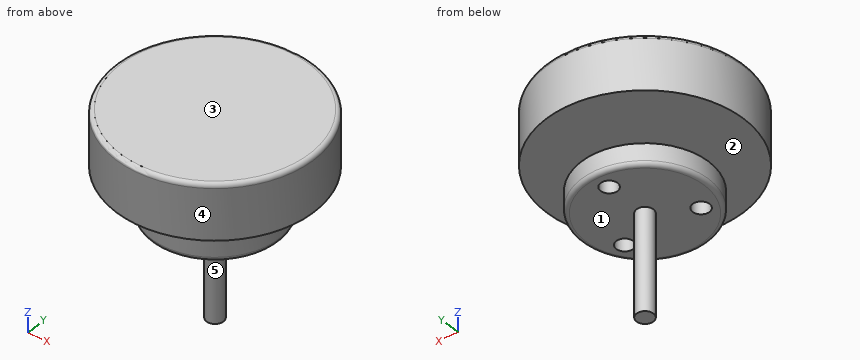
```python
from build123d import *

# Parameters (mm, degrees)
SKETCH1_R           = 11.65
BOSS_EXTRUDE1_DEPTH = 6.5
FILLET1_R           = 0.5
SKETCH2_R           = 3.25
BOSS_EXTRUDE2_DEPTH = 3
SKETCH3_R           = 7.5
BOSS_EXTRUDE3_DEPTH = 2.5
FILLET2_R           = 0.5
SKETCH4_R           = 1
BOSS_EXTRUDE4_DEPTH = 12
CUT_EXTRUDE1_REACH  = 22.382
SKETCH5_R           = 1


with BuildPart() as part:
    # Sketch1 → Boss-Extrude1 (new body)
    with BuildSketch(Plane.XY):
        with Locations(Location((0, 0, 0), (0, 0, 180))):
            Circle(SKETCH1_R)
    extrude(amount=BOSS_EXTRUDE1_DEPTH)

    # Fillet1
    fillet1_edges = [part.edges().sort_by_distance(p)[0] for p in [
        (11.65, 0, 6.5),
    ]]
    fillet(fillet1_edges, radius=FILLET1_R)

    # Sketch2 → Boss-Extrude2 (add)
    with BuildSketch(Plane(origin=(0, 0, 0), x_dir=(-1, 0, 0), z_dir=(0, 0, -1))):
        Circle(SKETCH2_R)
    extrude(amount=BOSS_EXTRUDE2_DEPTH)

    # Sketch3 → Boss-Extrude3 (add)
    with BuildSketch(Plane(origin=(0, 0, -3), x_dir=(-1, 0, 0), z_dir=(0, 0, -1))):
        Circle(SKETCH3_R)
    extrude(amount=BOSS_EXTRUDE3_DEPTH)

    # Fillet2
    fillet2_edges = [part.edges().sort_by_distance(p)[0] for p in [
        (7.5, 0, -5.5),
    ]]
    fillet(fillet2_edges, radius=FILLET2_R)

    # Sketch4 → Boss-Extrude4 (add)
    with BuildSketch(Plane(origin=(0, 0, -5.5), x_dir=(-1, 0, 0), z_dir=(0, 0, -1))):
        Circle(SKETCH4_R)
    extrude(amount=BOSS_EXTRUDE4_DEPTH)

    # Sketch5 → Cut-Extrude1 (cut, up to next)
    with BuildSketch(Plane(origin=(0, 0, -5.5), x_dir=(-1, 0, 0), z_dir=(0, 0, -1)), mode=Mode.PRIVATE) as cut_extrude1_sk1:
        with Locations((4.54663337, -2.625)):
            Circle(SKETCH5_R)
    cut_extrude1_tool1 = extrude(cut_extrude1_sk1.sketch, amount=-CUT_EXTRUDE1_REACH, mode=Mode.PRIVATE) & part.part
    # Sketch5 → Cut-Extrude1 (cut, up to next)
    with BuildSketch(Plane(origin=(0, 0, -5.5), x_dir=(-1, 0, 0), z_dir=(0, 0, -1)), mode=Mode.PRIVATE) as cut_extrude1_sk2:
        with Locations((0, 5.25)):
            Circle(SKETCH5_R)
    cut_extrude1_tool2 = extrude(cut_extrude1_sk2.sketch, amount=-CUT_EXTRUDE1_REACH, mode=Mode.PRIVATE) & part.part
    # Sketch5 → Cut-Extrude1 (cut, up to next)
    with BuildSketch(Plane(origin=(0, 0, -5.5), x_dir=(-1, 0, 0), z_dir=(0, 0, -1)), mode=Mode.PRIVATE) as cut_extrude1_sk3:
        with Locations((-4.54663337, -2.625)):
            Circle(SKETCH5_R)
    cut_extrude1_tool3 = extrude(cut_extrude1_sk3.sketch, amount=-CUT_EXTRUDE1_REACH, mode=Mode.PRIVATE) & part.part
    add(cut_extrude1_tool1.solids().sort_by_distance((-4.546633, -2.625, -5.5))[0], mode=Mode.SUBTRACT)
    add(cut_extrude1_tool2.solids().sort_by_distance((0, 5.25, -5.5))[0], mode=Mode.SUBTRACT)
    add(cut_extrude1_tool3.solids().sort_by_distance((4.546633, -2.625, -5.5))[0], mode=Mode.SUBTRACT)


solid = part.part
```
Input: part model. Units: mm. Frame: model coordinates. Face numbers are marked on the shaded views. A direction names the side the tool comes from. Give positions to 0.01 mm unless a question says otherwise; leave off trailing zeros. Loops run counter-clockwise (first coordinate to the right, second up) from the corner with the lowest first, then second, coordinate; pieces in that order, holes last. Notation, with made-up numbers: M 76,52 L 114,52 A31 cw 114,83 Z; hole C 40.5,32 d10. An arc over 180 degrees is marked long. Answer as CSV lines item,"result". Start each with the question number.
1. Section D-D on y = 5.25. State how many separate pieces and enclosed holes the cut face has, plus the area to 3 significant figures.
2. Section A-A on x = 0. Return loops of the section in (y, z).
3. Reachability of the marked faces 4 and 5 from +Z, -Z, +X, -X, +Y, -Y: full face, straight path, thin tool, end or side. Return the list, or none.
4. Pull-direction query (Z, two-part tool) for the marked faces 1, 2 and 3; classes: released by +Z, released by -Z, zero draft, split by the parting line, or undercut.
5. Section B-B on y = 0. Return loops of the section in (x, z), plus the area to 3 significant figures.
6. Section C-C on z = 1.5. Return loops of the section in (x, y).
7. Line query: L1, parallel to Y at x = 0, z = -4; L2, parallel to Z at x = -5.25, y = 6.25; L3, parallel to X at y = 5.5, z = -3.5. Output: solid intervals per line, ascending.
8. Pin query (flat end, axial travel): P1, Ø4, axis at y = 6.5, z = -2.5, coming from the -X side; P2, Ø5, axis at x = -1.5, z = -14.5, coming from the -Y side; P3, Ø1, axis at y = -6, z = -4, coming from the -X side. Return the tip coordinate at first contact, or that it passes through.
Computed values:
1,separate pieces,"3"
1,enclosed holes,"0"
1,area,"157 mm²"
2,outline,"M -11.65,0 L -3.25,0 L -3.25,-3 L -7.5,-3 L -7.5,-5 A0.5 ccw -7,-5.5 L -1,-5.5 L -1,-17.5 L 1,-17.5 L 1,-5.5 L 4.25,-5.5 L 4.25,-3 L 3.25,-3 L 3.25,0 L 11.65,0 L 11.65,6 A0.5 ccw 11.15,6.5 L -11.15,6.5 A0.5 ccw -11.65,6 Z; M 6.25,-5.5 L 7,-5.5 A0.5 ccw 7.5,-5 L 7.5,-3 L 6.25,-3 Z"
3,face 4,"+Z, -Z"
3,face 5,"-Z"
4,face 1,"released by -Z"
4,face 2,"undercut"
4,face 3,"released by +Z"
5,outline,"M -11.65,0 L -3.25,0 L -3.25,-3 L -7.5,-3 L -7.5,-5 A0.5 ccw -7,-5.5 L -1,-5.5 L -1,-17.5 L 1,-17.5 L 1,-5.5 L 7,-5.5 A0.5 ccw 7.5,-5 L 7.5,-3 L 3.25,-3 L 3.25,0 L 11.65,0 L 11.65,6 A0.5 ccw 11.15,6.5 L -11.15,6.5 A0.5 ccw -11.65,6 Z"
5,area,"232 mm²"
6,outline,"C 0,0 d23.3"
7,L1,"y = -7.5 to 4.25, 6.25 to 7.5"
7,L2,"z = 0 to 6.5"
7,L3,"x = -5.1 to -0.97, 0.97 to 5.1"
8,P1,"stops at x = -5.95"
8,P2,"stops at y = -1"
8,P3,"stops at x = -5.1"
